Geometry: final body of the model. Coordinates: model frame, mm. A direction names the side the tool comes from. Give positions to 0.01 mm unless a question says otherwise; leave off trailing zeros. Order: outer loops, then holes, each group sorted by start corner. A loop starts at its lowest first (then second) coordinate and runs counter-clockwise, first axis right, second up. Notation, with made-up numbers: (77.5, -29) -> (118.5, -29) arc R19 cw to (118.5, -21) -> close; hole circle Ø2 at (4.5, 20.5). An arc over 180 degrees is marked (long way). Answer in a Markdown table with one row per item. Add a question column.
Q1. Cut plane B-B on y = 13. Return the cut outline in (x, z).
Q2. Cut plane D-D on y = 7. Return the cut outline in (x, z), and give its area (3 significant figures).
Q3. Set-up query: faces 1 (the face through (-0.5, 3.4, -12.3)), 2 (the face through (-3.4, 0.5, -12.3)), 3 (the face through (-0.5, -3.4, -12.3)). Return all of +Z, -Z, +X, -X, +Y, -Y with unobstructed straight access to the full face (end or side cutting, diameter ignored); none if empty.
Q4. Line query: line 1 along X through (y, z) = (-2.5, -15.5); line 2 along Y through (x, z) = (3, -8); line 3 along Z through (x, y) = (5, -13.5). Output: solid intervals per line, ascending. Write a range as from..to.
Q5. Pull-direction query (Y, two-part tool) for faces 4 (the face through (0.5, -3.4, -12.3)), 5 (the face through (-2.72, -1.14, -12.32)), 6 (the face through (15.29, -16.64, 1.97)), 7 (the face through (0, 4, -12)); classes: +Y half, -Y half, draft (parallel to the pull), parting line (faces both ways), or undercut.
Q6. Contact query for flat-ended pins moving along their axis: P1, Ø6, axis at x = 1, z = -2.5, coming from the -Y side; P2, Ø0.5, axis at y = 3.5, z = -16.5, coming from the +X side; P3, Ø0.5, axis at y = -3.5, z = -10, coming from the -X side; P4, Ø0.5, axis at x = -3.5, z = -9.5, coming from the +Y side. Output: stop coordinate, or through.
Q7. Cut plane A-A on x = -16. Return the cut outline in (y, z), and give its area (3 significant figures).
from build123d import *

# Parameters (mm, degrees)
F0_W     = 40
F0_H     = 40
F0_R     = 3.175
F1_DEPTH = 4
F3_DEPTH = 25


with BuildPart() as f1:
    # F0 (on Top) → F1 (new body)
    with BuildSketch(Plane.XY):
        Rectangle(F0_W, F0_H)
        with Locations((-13.825, -13.825)):
            Circle(F0_R, mode=Mode.SUBTRACT)
        with Locations((13.825, -13.825)):
            Circle(F0_R, mode=Mode.SUBTRACT)
        with Locations((-13.825, 13.825)):
            Circle(F0_R, mode=Mode.SUBTRACT)
        with Locations((13.825, 13.825)):
            Circle(F0_R, mode=Mode.SUBTRACT)
    extrude(amount=F1_DEPTH)

    # F2 (on face) → F3 (join)
    with BuildSketch(Plane(origin=(0, 0, 0), x_dir=(1, 0, 0), z_dir=(0, 0, -1))):
        with BuildLine():
            ThreePointArc((1.702231, 2.409338), (2.085965, 2.085965), (2.409338, 1.702231))
            Line((2.409338, 1.702231), (3.159796, 2.45269))
            ThreePointArc((3.159796, 2.45269), (2.828427, 2.828427), (2.45269, 3.159796))
            Line((2.45269, 3.159796), (1.702231, 2.409338))
        make_face()
        with BuildLine():
            ThreePointArc((-0.5, 2.907318), (0, 2.95), (0.5, 2.907318))
            Line((0.5, 2.907318), (0.5, 3.968627))
            ThreePointArc((0.5, 3.968627), (0, 4), (-0.5, 3.968627))
            Line((-0.5, 3.968627), (-0.5, 2.907318))
        make_face()
        with BuildLine():
            ThreePointArc((-2.409338, 1.702231), (-2.085965, 2.085965), (-1.702231, 2.409338))
            Line((-1.702231, 2.409338), (-2.45269, 3.159796))
            ThreePointArc((-2.45269, 3.159796), (-2.828427, 2.828427), (-3.159796, 2.45269))
            Line((-3.159796, 2.45269), (-2.409338, 1.702231))
        make_face()
        with BuildLine():
            ThreePointArc((-2.907318, -0.5), (-2.95, 0), (-2.907318, 0.5))
            Line((-2.907318, 0.5), (-3.968627, 0.5))
            ThreePointArc((-3.968627, 0.5), (-4, 0), (-3.968627, -0.5))
            Line((-3.968627, -0.5), (-2.907318, -0.5))
        make_face()
        with BuildLine():
            Line((-2.45269, -3.159796), (-1.702231, -2.409338))
            ThreePointArc((-1.702231, -2.409338), (-2.085965, -2.085965), (-2.409338, -1.702231))
            Line((-2.409338, -1.702231), (-3.159796, -2.45269))
            ThreePointArc((-3.159796, -2.45269), (-2.828427, -2.828427), (-2.45269, -3.159796))
        make_face()
        with BuildLine():
            Line((0.5, -3.968627), (0.5, -2.907318))
            ThreePointArc((0.5, -2.907318), (0, -2.95), (-0.5, -2.907318))
            Line((-0.5, -2.907318), (-0.5, -3.968627))
            ThreePointArc((-0.5, -3.968627), (0, -4), (0.5, -3.968627))
        make_face()
        with BuildLine():
            Line((3.159796, -2.45269), (2.409338, -1.702231))
            ThreePointArc((2.409338, -1.702231), (2.085965, -2.085965), (1.702231, -2.409338))
            Line((1.702231, -2.409338), (2.45269, -3.159796))
            ThreePointArc((2.45269, -3.159796), (2.828427, -2.828427), (3.159796, -2.45269))
        make_face()
        with BuildLine():
            ThreePointArc((2.907318, 0.5), (2.93931, 0.250909), (2.95, 0))
            ThreePointArc((2.95, 0), (2.93931, -0.250909), (2.907318, -0.5))
            Line((2.907318, -0.5), (3.968627, -0.5))
            ThreePointArc((3.968627, -0.5), (3.992149, -0.250492), (4, 0))
            ThreePointArc((4, 0), (3.992149, 0.250492), (3.968627, 0.5))
            Line((3.968627, 0.5), (2.907318, 0.5))
        make_face()
        with BuildLine():
            ThreePointArc((2.907318, -0.5), (2.93931, -0.250909), (2.95, 0))
            ThreePointArc((2.95, 0), (2.93931, 0.250909), (2.907318, 0.5))
            ThreePointArc((2.907318, 0.5), (2.725445, 1.128916), (2.409338, 1.702231))
            ThreePointArc((2.409338, 1.702231), (2.085965, 2.085965), (1.702231, 2.409338))
            ThreePointArc((1.702231, 2.409338), (1.128916, 2.725445), (0.5, 2.907318))
            ThreePointArc((0.5, 2.907318), (0, 2.95), (-0.5, 2.907318))
            ThreePointArc((-0.5, 2.907318), (-1.128916, 2.725445), (-1.702231, 2.409338))
            ThreePointArc((-1.702231, 2.409338), (-2.085965, 2.085965), (-2.409338, 1.702231))
            ThreePointArc((-2.409338, 1.702231), (-2.725445, 1.128916), (-2.907318, 0.5))
            ThreePointArc((-2.907318, 0.5), (-2.95, 0), (-2.907318, -0.5))
            ThreePointArc((-2.907318, -0.5), (-2.725445, -1.128916), (-2.409338, -1.702231))
            ThreePointArc((-2.409338, -1.702231), (-2.085965, -2.085965), (-1.702231, -2.409338))
            ThreePointArc((-1.702231, -2.409338), (-1.128916, -2.725445), (-0.5, -2.907318))
            ThreePointArc((-0.5, -2.907318), (0, -2.95), (0.5, -2.907318))
            ThreePointArc((0.5, -2.907318), (1.128916, -2.725445), (1.702231, -2.409338))
            ThreePointArc((1.702231, -2.409338), (2.085965, -2.085965), (2.409338, -1.702231))
            ThreePointArc((2.409338, -1.702231), (2.725445, -1.128916), (2.907318, -0.5))
        make_face()
    extrude(amount=F3_DEPTH)


solid = f1.part
Completed:
| question | item | result |
|---|---|---|
| 1 | outline | (-20, 0) -> (-16.89, 0) -> (-16.89, 4) -> (-20, 4) -> close; (-10.76, 0) -> (10.76, 0) -> (10.76, 4) -> (-10.76, 4) -> close; (16.89, 0) -> (20, 0) -> (20, 4) -> (16.89, 4) -> close |
| 2 | outline | (-20, 0) -> (20, 0) -> (20, 4) -> (-20, 4) -> close |
| 2 | area | 160 mm² |
| 3 | face 1 | -Z, +Y |
| 3 | face 2 | -Z, -X |
| 3 | face 3 | -Z, -Y |
| 4 | line 1 | x = -3.12..-1.79, -1.57..1.57, 1.79..3.12 |
| 4 | line 2 | y = -2.65..-2.29, -0.5..0.5, 2.29..2.65 |
| 4 | line 3 | z = 0..4 |
| 5 | face 4 | draft |
| 5 | face 5 | undercut |
| 5 | face 6 | undercut |
| 5 | face 7 | +Y half |
| 6 | P1 | stops at y = -20 |
| 6 | P2 | stops at x = 0.5 |
| 6 | P3 | stops at x = -0.5 |
| 6 | P4 | stops at y = 0.5 |
| 7 | outline | (-20, 0) -> (-16.14, 0) -> (-16.14, 4) -> (-20, 4) -> close; (-11.51, 0) -> (11.51, 0) -> (11.51, 4) -> (-11.51, 4) -> close; (16.14, 0) -> (20, 0) -> (20, 4) -> (16.14, 4) -> close |
| 7 | area | 123 mm² |
